Autodesk Inventor part; units mm, degrees
ref_plane "YZ Plane" through (0, 0, 0) normal (1, 0, 0) x (0, 1, 0)
ref_plane "XZ Plane" through (0, 0, 0) normal (0, 1, 0) x (-1, 0, 0)
ref_plane "XY Plane" through (0, 0, 0) normal (0, 0, 1) x (1, 0, 0)
sketch "草圖1" plane through (0, 0, 0) normal (0, 0, 1) x (1, 0, 0)
  line L0 (-348.7345, 0) -> (348.7345, 0)
  line L1 (348.7345, 0) -> (348.7345, -20)
  line L2 (348.7345, -20) -> (-348.7345, -20)
  line L3 (-348.7345, -20) -> (-348.7345, 0)
  line L4 (-348.7345, 0) -> (-358.7345, 0)
  line L5 (-358.7345, 0) -> (-358.7345, -10)
  line L6 (-358.7345, -10) -> (-348.7345, -10)
  line L7 (-348.7345, -10) -> (-348.7345, 0)
  line L8 (348.7345, 0) -> (358.7345, 0)
  line L9 (358.7345, 0) -> (358.7345, -10)
  line L10 (358.7345, -10) -> (348.7345, -10)
  line L11 (348.7345, -10) -> (348.7345, 0)
  point P0 (0, 0)
  point P1 (0, 0)
  dimension "d0" = 697.469
  dimension "d1" = 40
  dimension "d2" = 20
  dimension "d3" = 10
  dimension "d4" = 20
  dimension "d5" = 10
revolve "迴轉1" add sketch "草圖1" angle 360 about axis through (-348.7345, 0, 0) along (1, 0, 0)
sketch "草圖2" plane through (0, 0, 0) normal (0, 0, 1) x (1, 0, 0)
  line L0 (358.7345, 10) -> (358.7345, -10) construction
  line L1 (358.7345, -10) -> (348.7345, -10) construction
  line L2 (348.7345, -10) -> (348.7345, -20) construction
  line L3 (348.7345, -20) -> (-348.7345, -20) construction
  line L4 (-348.7345, -20) -> (-348.7345, -10) construction
  line L5 (-348.7345, -10) -> (-358.7345, -10) construction
  line L6 (-358.7345, -10) -> (-358.7345, 10) construction
  line L7 (-358.7345, 10) -> (-348.7345, 10) construction
  line L8 (-348.7345, 10) -> (-348.7345, 20) construction
  line L9 (-348.7345, 20) -> (348.7345, 20) construction
  line L10 (348.7345, 20) -> (348.7345, 10) construction
  line L11 (348.7345, 10) -> (358.7345, 10) construction
  line L12 (348.7345, -20) -> (348.7345, -342.9396) construction
  line L13 (346.2345, -215) -> (348.7345, -215)
  line L14 (348.7345, -215) -> (348.7345, -20)
  line L15 (348.7345, -20) -> (346.2345, -20)
  line L16 (346.2345, -20) -> (346.2345, -215)
  line L17 (358.7345, -10) -> (348.7345, -10) construction
  line L18 (348.7345, -10) -> (348.7345, -20) construction
  line L19 (348.7345, -20) -> (-348.7345, -20) construction
  line L20 (-348.7345, -20) -> (-348.7345, -10) construction
  line L21 (-348.7345, -10) -> (-358.7345, -10) construction
  line L22 (-358.7345, 10) -> (-348.7345, 10) construction
  line L23 (-348.7345, 10) -> (-348.7345, 20) construction
  line L24 (-348.7345, 20) -> (348.7345, 20) construction
  line L25 (348.7345, 20) -> (348.7345, 10) construction
  line L26 (348.7345, 10) -> (358.7345, 10) construction
  line L27 (358.7345, 10) -> (358.7345, -10)
  line L28 (-358.7345, -10) -> (-358.7345, 10)
  point P0 (0, 0)
  dimension "d9" = 2.5
  dimension "d10" = 215
coil "螺旋1" sketch "草圖2" operation add axis through (-10, 0, 0) along (-1, 0, 0) pitch 173.5 turns 4 hand left
equation "\"d4\" = d2"
equation "\"d5\" = d3"
properties part number "Screw shaft"
The listing builds one solid part. Answer for the finished solid, in the listing's coordinates (mm). A direction names the side the tool comes from. Coordinates: 2 decimals unless noted, no trailing zeros. Write item = value, one per line. Start each with the question number.
1) Straight lines are drawn through the part: line 1 (X direction, y = -169, z = -54); line 2 (X direction, y = 79.5, z = -27.5); line 3 (Y direction, x = -187.5, z = -3). For each, find the intervals that lie inside material, in ascending order. Write a range as from..to.
2) A cutting plane is placed at A-A (z = 145). Count the separate pieces of the cut face and the enclosed holes in it, then the cut area to 3 significant figures.
3) A tool of negligible diameter and unlimited length cuts with its end or side. For faces 1 (the face through (353.66, 2.17, -9.76)), 2 (the face through (-358.734, 0, 0)), 3 (the face through (-353.66, 2.17, 9.76)), from which of +Z, -Z, +X, -X, +Y, -Y can it reach the whole face along a straight path? Write none if from no direction.
4) Given pin 1 Ø2 at (x, z) = (138, -52) entering from +Y; pin 2 Ø2 at (x, y) = (347, -153) entering from +Z; pin 3 Ø10 at (y, z) = (-115.5, -90.5) entering from -X, each flat-ended and moving along its own axis, determine where each tip first touches the part or whether it passes through.
Responses:
q1.line_1 = -182.81..-180.31, -9.31..-6.81, 164.19..166.69, 337.69..340.19
q1.line_2 = -251.82..-249.32, -78.32..-75.82, 95.18..97.68, 268.68..271.18
q1.line_3 = -19.77..19.77
q2.separate_pieces = 4
q2.enclosed_holes = 0
q2.area = 3,170 mm²
q3.face_1 = +X
q3.face_2 = +Z, -Z, -X, +Y, -Y
q3.face_3 = -X
q4.pin_1 = -9.78
q4.pin_2 = 0
q4.pin_3 = -193.56
